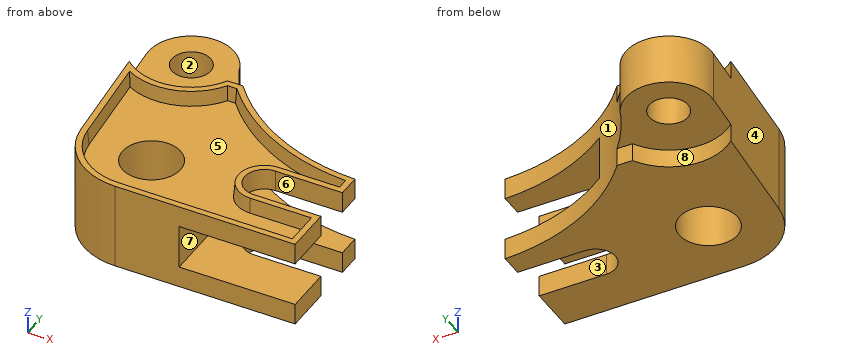
```python
from build123d import *

# Parameters (mm, degrees)
ESQUISSE1_R             = 6.35
ESQUISSE1_R_2           = 9.5
BOSS_EXTRU_1_DEPTH      = 28.5
ENL_V_START             = -6
ENL_V_MAT_EXTRU_1_DEPTH = 6
ENL_V_MAT_EXTRU_2_DEPTH = 6
ESQUISSE4_W             = 38
ESQUISSE4_H             = 14.5
ENL_V_MAT_EXTRU_3_DEPTH = 124.584469767
ENL_V_MAT_EXTRU_5_DEPTH = 5
ENL_V_MAT_EXTRU_5_DRAFT = -5


with BuildPart() as part:
    # Esquisse1 → Boss.-Extru.1 (new body)
    with BuildSketch(Plane.XY):
        with BuildLine():
            Line((-86.633280406, -6.99307262), (-81.912918385, -55.104590809))
            ThreePointArc((-81.912918385, -55.104590809), (-74.795399572, -69.254576275), (-60.018047616, -74.956420883))
            Line((-60.018047616, -74.956420883), (-1.018047616, -74.956420883))
            Line((-1.018047616, -74.956420883), (-1.018047616, -59.456420883))
            Line((-1.018047616, -59.456420883), (-23.018047616, -59.456420883))
            ThreePointArc((-23.018047616, -59.456420883), (-29.518047616, -52.956420883), (-23.018047616, -46.456420883))
            Line((-23.018047616, -46.456420883), (-1.018047616, -46.456420883))
            Line((-1.018047616, -46.456420883), (-1.018047616, -38.956420883))
            ThreePointArc((-1.018047616, -38.956420883), (-35.318453229, -28.420111536), (-59.263146108, -1.695902984))
            ThreePointArc((-59.263146108, -1.695902984), (-75.360354059, 8.118888343), (-86.633280406, -6.99307262))
        make_face()
        with Locations(Location((-72.700180587, -5.626055331, 0), (0, 0, 180))):
            Circle(ESQUISSE1_R, mode=Mode.SUBTRACT)
        with Locations(Location((-60.018047616, -52.956420883, 0), (0, 0, 180))):
            Circle(ESQUISSE1_R_2, mode=Mode.SUBTRACT)
    extrude(amount=BOSS_EXTRU_1_DEPTH)

    # Esquisse2 → Enlèv. mat.-Extru.1 (cut)
    with BuildSketch(Plane.XY.offset(28.5).offset(ENL_V_START)):
        with BuildLine():
            Line((-50.888781824, -14.626055395), (-55.966980296, -14.626055395))
            ThreePointArc((-55.966980296, -14.626055395), (-69.422632675, -24.341227799), (-85.379019392, -19.776922952))
            Line((-85.379019392, -19.776922952), (-86.633280406, -6.99307262))
            ThreePointArc((-86.633280406, -6.99307262), (-75.360354059, 8.118888343), (-59.263146108, -1.695902984))
            ThreePointArc((-59.263146108, -1.695902984), (-55.448825079, -8.402467045), (-50.888781824, -14.626055395))
        make_face()
    extrude(amount=ENL_V_MAT_EXTRU_1_DEPTH, mode=Mode.SUBTRACT)

    # Esquisse3 → Enlèv. mat.-Extru.2 (cut)
    with BuildSketch(Plane(origin=(0, 0, 0), x_dir=(-1, 0, 0), z_dir=(0, 0, -1))):
        with BuildLine():
            Line((85.379019392, -19.776922952), (86.633280406, -6.99307262))
            ThreePointArc((86.633280406, -6.99307262), (75.360354059, 8.118888343), (59.263146108, -1.695902984))
            ThreePointArc((59.263146108, -1.695902984), (55.448825079, -8.402467045), (50.888781824, -14.626055395))
            Line((50.888781824, -14.626055395), (55.966980296, -14.626055395))
            ThreePointArc((55.966980296, -14.626055395), (69.422632675, -24.341227799), (85.379019392, -19.776922952))
        make_face()
    extrude(amount=-ENL_V_MAT_EXTRU_2_DEPTH, mode=Mode.SUBTRACT)

    # Esquisse4 → Enlèv. mat.-Extru.3 (cut, through all)
    with BuildSketch(Plane.XZ.offset(74.956420883)):
        with Locations((-20.018047616, 14.25)):
            Rectangle(ESQUISSE4_W, ESQUISSE4_H)
    extrude(amount=-ENL_V_MAT_EXTRU_3_DEPTH, mode=Mode.SUBTRACT)


with BuildPart() as enl_v_mat_extru_5_tool:
    # Esquisse5 → Enlèv. mat.-Extru.5 (with draft: the straight prism first)
    with BuildSketch(Plane.XY.offset(28.5)):
        with BuildLine():
            Line((-51.822935649, -16.626055395), (-54.811637006, -16.626055395))
            ThreePointArc((-54.811637006, -16.626055395), (-67.412845938, -25.949541557), (-82.960069876, -23.949119459))
            Line((-82.960069876, -23.949119459), (-79.922475588, -54.909302634))
            ThreePointArc((-79.922475588, -54.909302634), (-73.452003939, -67.772925785), (-60.018047616, -72.956420883))
            Line((-60.018047616, -72.956420883), (-3.018047616, -72.956420883))
            Line((-3.018047616, -72.956420883), (-3.018047616, -61.456420883))
            Line((-3.018047616, -61.456420883), (-23.018047616, -61.456420883))
            ThreePointArc((-23.018047616, -61.456420883), (-31.518047616, -52.956420883), (-23.018047616, -44.456420883))
            Line((-23.018047616, -44.456420883), (-3.018047616, -44.456420883))
            Line((-3.018047616, -44.456420883), (-3.018047616, -40.875747076))
            ThreePointArc((-3.018047616, -40.875747076), (-29.916011773, -33.773380805), (-51.822935649, -16.626055395))
        make_face()
    extrude(amount=-ENL_V_MAT_EXTRU_5_DEPTH)
    # Enlèv. mat.-Extru.5: the draft: its side faces are tilted about the plane it starts from
    enl_v_mat_extru_5_sides = [enl_v_mat_extru_5_tool.faces().sort_by_distance(p)[0] for p in [
        (-53.317286327, -16.626055395, 26),
        (-67.412845938, -25.949541557, 26),
        (-81.441272732, -39.429211046, 26),
        (-73.452003939, -67.772925785, 26),
        (-31.518047616, -72.956420883, 26),
        (-3.018047616, -67.206420883, 26),
        (-13.018047616, -61.456420883, 26),
        (-31.518047616, -52.956420883, 26),
        (-13.018047616, -44.456420883, 26),
        (-3.018047616, -42.66608398, 26),
        (-29.916011773, -33.773380805, 26),
    ]]
    draft(enl_v_mat_extru_5_sides, Plane.XY.offset(28.5), ENL_V_MAT_EXTRU_5_DRAFT)


with BuildPart() as part_1:
    add(part.part)

    # Enlèv. mat.-Extru.5: cut by enl_v_mat_extru_5_tool
    add(enl_v_mat_extru_5_tool.part, mode=Mode.SUBTRACT)


solid = part_1.part
```
Here's how the part is built. I have some questions about the finished solid (model axes, mm). Face numbers are marked on the shaded views. A direction names the side the tool comes from. Coordinates: 2 decimals unless noted, no trailing zeros. Loops run counter-clockwise (first coordinate to the right, second up) from the corner with the lowest first, then second, coordinate; pieces in that order, holes last. Notation, with made-up numbers: (38.5, -7.5) - (61.5, -7.5) arc R34 cw to (61.5, 30.5) - close; hole circle Ø5 at (14, -0.75). An arc over 180 degrees is marked (long way). Return JSON: item names as keys, results as strings. Group by question number.
Item 1: On a 3-axis mill with a long thin cutter (end or side, diameter ignored), from which of +Z, -Z, +X, -X, +Y, -Y can I reach the whole of each face in a straight line? I mean the marked faces 5, 6, 7 and 8. Say none if no direction works.
Item 2: If we section it at D-D on x = -8.5: State how many separate pieces and enclosed holes the cut face has, and give its area (3 significant figures).
Item 3: Will these pins go through, and if not, where does the flat tip stop? P1, Ø12, axis at y = -28.5, z = 20.5, coming from the -X side; P2, Ø12, axis at x = -34, y = -32.5, coming from the +Z side; P3, Ø2, axis at x = -17, z = 4, coming from the +Y side; P4, Ø4, axis at x = -50.5, z = 5.5, coming from the +Y side.
Item 4: If we section it at A-A on y = -4: Write out the boundary of the cut face in (x, z).
Item 5: I need wall thicknesses on line 1 (Z direction, x = -38, y = -37.5); line 2 (Z direction, x = -56.5, y = -66); line 3 (Y direction, x = -77, z = 20.75). Which ranges of each line are inside material? Lowest first, please. Write a range as from..to.
Item 6: If we section it at C-C on z = 2.75: Write out the boundary of the cut face in (x, y).
Item 7: We'd pull the mould along X, two halves only. Please class the marked faces 1, 2, 3 and 4: +X half, -X half, draft (parallel to the pull), parting line (faces both ways), or undercut.
Item 8: If we section it at B-B on z = 16: Write out the boundary of the cut face in (x, y).
Calculated:
{
 "1": {"face 5": "+Z", "face 6": "+Z, -Z, +X", "face 7": "+X, +Y, -Y", "face 8": "-Z, +Y"},
 "2": {"separate pieces": "4", "enclosed holes": "0", "area": "257 mm^2"},
 "3": {"P1": "stops at x = -85.11", "P2": "stops at z = 28.5", "P3": "stops at y = -36.29", "P4": "stops at y = -12.68"},
 "4": {"outline": "(-86.61, 6) - (-78.84, 6) - (-78.84, 22.5) - (-86.61, 22.5) - close; (-66.56, 6) - (-58.07, 6) - (-58.07, 22.5) - (-66.56, 22.5) - close"},
 "5": {"line 1": "z = 0..7, 21.5..23.5", "line 2": "z = 0..23.5", "line 3": "y = -66.94..-10.3, -0.95..7.7"},
 "6": {"outline": "(-85.38, -19.78) - (-81.91, -55.1) arc R22 ccw to (-60.02, -74.96) - (-1.02, -74.96) - (-1.02, -59.46) - (-23.02, -59.46) arc R6.5 cw to (-23.02, -46.46) - (-1.02, -46.46) - (-1.02, -38.96) arc R67 cw to (-50.89, -14.63) - (-55.97, -14.63) arc R19 cw to start; hole circle Ø19 at (-60.02, -52.96)"},
 "7": {"face 1": "+X half", "face 2": "undercut", "face 3": "draft", "face 4": "-X half"},
 "8": {"outline": "(-86.63, -6.99) - (-81.91, -55.1) arc R22 ccw to (-60.02, -74.96) - (-39.02, -74.96) - (-39.02, -25.87) arc R67 cw to (-59.26, -1.7) arc R14 ccw to start; hole circle Ø12.7 at (-72.7, -5.63); hole circle Ø19 at (-60.02, -52.96)"}
}
